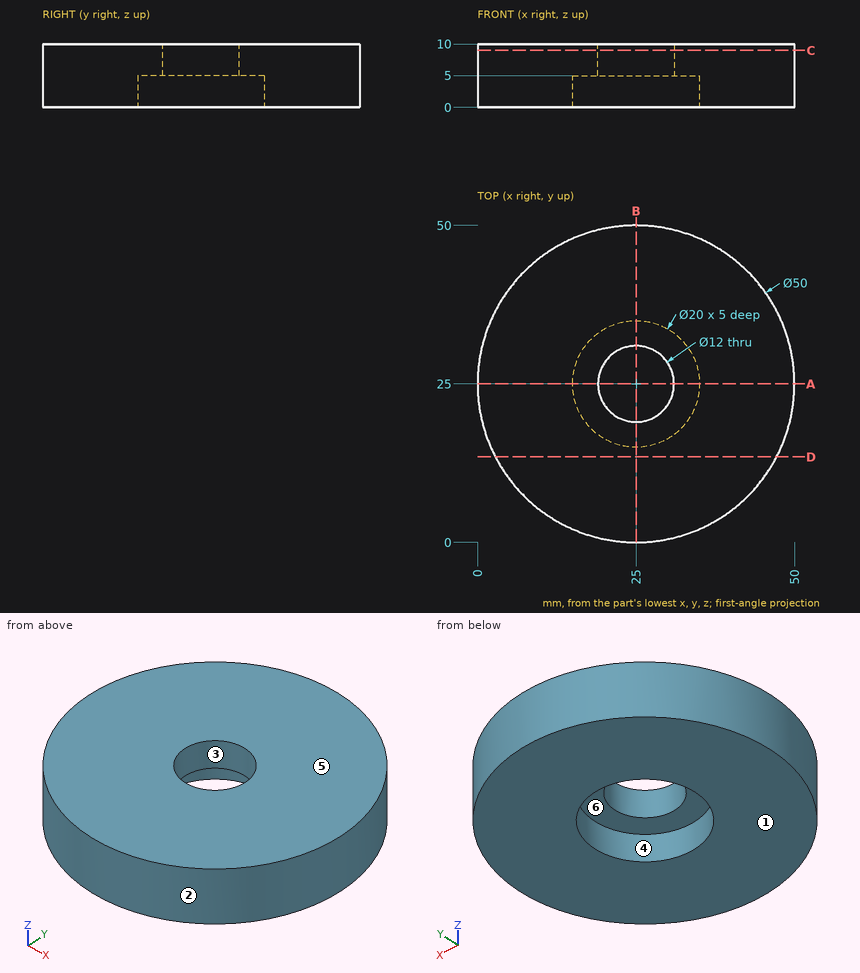
Can you work these out from the drawing? Everything is in mm from the part's minimum corner. A direction names the side the tool comes from. Coordinates: 2 decimals unless noted, no trailing zeros. Loops run counter-clockwise (first coordinate to the right, second up) from the corner with the lowest first, then second, coordinate; pieces in that order, holes last.
1. I need wall thicknesses on L1, parallel to Y at x = 25, z = 8; L2, parallel to Y at x = 25, z = 3.85; L3, parallel to Z at x = 25, y = 16.5. Which ranges of each line are inside material? Lowest first, please.
2. For P1, Ø3, axis at y = 42, z = 2, coming from the +X side; P2, Ø4, axis at y = 39.5, z = 7, coming from the -X side; P3, Ø3, axis at y = 18, z = 2.5, coming from the -X side, each with a flat end and sliding along its axis, tell me the tip position at first contact or that it passes through.
3. Imagine slicing it at C-C, the plane z = 9. Please give me the cut outline in (x, y), and give its area (3 significant figures).
4. Imagine slicing it at D-D, the plane y = 13.5. Please give me the cut outline in (x, z).
5. For the marked faces 5 and 6, which set-ups out of +Z, -Z, +X, -X, +Y, -Y let a thin tool reach every point of the face, with its end or its side?
6. If we mould it in two halves opening along X, with no side actions, what happens to the marked faces 1, 2, 3 and 4? For each: pulls with the +X half, pulls with the -X half, needs draft (parallel to the pull), parting line crosses it, or undercut.
7. Imagine slicing it at A-A, the plane y = 25. Please give me the cut outline in (x, z), and give its area (3 significant figures).
Taken from the geometry:
1. L1: y = 0 to 19, 31 to 50
1. L2: y = 0 to 15, 35 to 50
1. L3: z = 5 to 10
2. P1: stops at x = 44.62
2. P2: stops at x = 3.35
2. P3: stops at x = 0.61
3. outline: circle Ø50 at (25, 25); hole circle Ø12 at (25, 25)
3. area: 1,850 mm2
4. outline: (2.8, 0) - (47.2, 0) - (47.2, 10) - (2.8, 10) - close
5. face 5: +Z, +X, -X, +Y, -Y
5. face 6: -Z
6. face 1: needs draft
6. face 2: parting line crosses it
6. face 3: undercut
6. face 4: undercut
7. outline: (0, 0) - (15, 0) - (15, 5) - (19, 5) - (19, 10) - (0, 10) - close; (31, 5) - (35, 5) - (35, 0) - (50, 0) - (50, 10) - (31, 10) - close
7. area: 340 mm2
